```python
from build123d import *

# Parameters (mm, degrees)
F0_W     = 50
F0_H     = 30
F1_DEPTH = 3
F2_W     = 5
F2_H     = 5
F3_DEPTH = 10
F4_R     = 1
F5_R     = 1
F6_R     = 1
F7_R     = 1


with BuildPart() as f1:
    # F0 (on Top) → F1 (new body)
    with BuildSketch(Plane.XY):
        with Locations((0, 5)):
            Rectangle(F0_W, F0_H)
    extrude(amount=F1_DEPTH)

    # F2 (on face) → F3 (join)
    with BuildSketch(Plane.XY.offset(3)):
        with Locations((-22.5, 17.5)):
            Rectangle(F2_W, F2_H)
        with Locations((22.5, 17.5)):
            Rectangle(F2_W, F2_H)
        with Locations((22.5, -7.5)):
            Rectangle(F2_W, F2_H)
        with Locations((-22.5, -7.5)):
            Rectangle(F2_W, F2_H)
    extrude(amount=F3_DEPTH)

    # F4
    f4_edges = [f1.edges().sort_by_distance(p)[0] for p in [
        (0, 20, 0),
    ]]
    fillet(f4_edges, radius=F4_R)

    # F5
    f5_edges = [f1.edges().sort_by_distance(p)[0] for p in [
        (25, 4.5, 0),
    ]]
    fillet(f5_edges, radius=F5_R)

    # F6
    f6_edges = [f1.edges().sort_by_distance(p)[0] for p in [
        (-0.5, -10, 0),
    ]]
    fillet(f6_edges, radius=F6_R)

    # F7
    f7_edges = [f1.edges().sort_by_distance(p)[0] for p in [
        (-25, 5, 0),
    ]]
    fillet(f7_edges, radius=F7_R)


solid = f1.part
```
Source: CAD feature listing. Evaluate the final solid. Frame: model axes, mm. A direction names the side the tool comes from. Coordinates: 2 decimals unless noted, no trailing zeros. Loops run counter-clockwise (first coordinate to the right, second up) from the corner with the lowest first, then second, coordinate; pieces in that order, holes last. Notation, with made-up numbers: M -24,26 L 27,26 A24 cw 27,58 Z; hole C 68.25,18.25 d1. An arc over 180 degrees is marked long. Use a Markdown table: item, result. Add a question column.
Q1. First-contact query: pin 1 (5 mm diameter, centred on x = -12, z = 4, fed in from -Y). Flat tip, straight axial feed; report the tip coordinate or a pass-through.
Q2. Section query A-A, the plane z = 8.5. Return loops of the section in (x, y), and give its area (3 significant figures).
Q3. Section query B-B, the plane y = 16.5. Return loops of the section in (x, z).
Q4. Section query C-C, the plane x = 6.5. Return loops of the section in (y, z), and give its area (3 significant figures).
Q5. Material intervals for L1, parallel to X at y = -6.5, z = 7; L2, parallel to Y at x = -22, z = 4; L3, parallel to Z at x = 10, y = -5.5, sorted ascending.
Q6. Section query D-D, the plane y = 7.25. Return loops of the section in (x, z).
Q7. Draft query along X for faces 4 (the cylindrical face through (0.336, 19.699, 0.285)), 5 (the flat face through (25, 5, 2)), 6 (the flat face through (-20, 17, 8)). Return one class per face: pulls with the +X half, pulls with the -X half, needs draft (parallel to the pull), parting line crosses it, or undercut.
Q8. Access query for faces 1 (the flat face through (22, -7, 13)), 2 (the flat face through (22, -5, 8)), 3 (the flat face through (20, -8, 8)). Directions: +Z, -Z, +X, -X, +Y, -Y. A direction counts if a zero-diameter tool reaches every point of the face in a straight line with its end or side. Return the directions, or none.
Result:
| question | item | result |
|---|---|---|
| 1 | pin 1 | stops at y = -10 |
| 2 | outline | M -25,-9 A1 ccw -24,-10 L -20,-10 L -20,-5 L -25,-5 Z; M -25,15 L -20,15 L -20,20 L -24,20 A1 ccw -25,19 Z; M 20,-10 L 24,-10 A1 ccw 25,-9 L 25,-5 L 20,-5 Z; M 20,15 L 25,15 L 25,19 A1 ccw 24,20 L 20,20 Z |
| 2 | area | 99.1 mm2 |
| 3 | outline | M -25,1 A1 ccw -24,0 L 24,0 A1 ccw 25,1 L 25,13 L 20,13 L 20,3 L -20,3 L -20,13 L -25,13 Z |
| 4 | outline | M -10,1 A1 ccw -9,0 L 19,0 A1 ccw 20,1 L 20,3 L -10,3 Z |
| 4 | area | 89.6 mm2 |
| 5 | L1 | x = -25 to -20, 20 to 25 |
| 5 | L2 | y = -10 to -5, 15 to 20 |
| 5 | L3 | z = 0 to 3 |
| 6 | outline | M -25,1 A1 ccw -24,0 L 24,0 A1 ccw 25,1 L 25,3 L -25,3 Z |
| 7 | face 4 | needs draft |
| 7 | face 5 | pulls with the +X half |
| 7 | face 6 | undercut |
| 8 | face 1 | +Z, +X, -X, +Y, -Y |
| 8 | face 2 | +Z, +X, -X |
| 8 | face 3 | +Z, +Y, -Y |
